```python
from build123d import *

# Parameters (mm, degrees)
BOX031_W     = 72
BOX031_H     = 58
BOX031_DEPTH = 4
FILLET025_R  = 10


with BuildPart() as fillet025:
    # Box031 → Box031 (new body)
    with BuildSketch(Plane(origin=(-15, -29, -2), x_dir=(1, 0, 0), z_dir=(0, 0, 1))):
        with Locations((36, 29)):
            Rectangle(BOX031_W, BOX031_H)
    extrude(amount=BOX031_DEPTH)

    # Fillet025
    fillet025_edges = [fillet025.edges().sort_by_distance(p)[0] for p in [
        (-15, -29, 0),
        (-15, 29, 0),
        (57, -29, 0),
        (57, 29, 0),
    ]]
    fillet(fillet025_edges, radius=FILLET025_R)


with BuildPart() as part_mirroring010:
    # Part__Mirroring010: instance of Fillet025
    add(fillet025.part.mirror(Plane(origin=(0, 0, 0), x_dir=(1, 0, 0), z_dir=(0, 1, 0))))


with BuildPart() as part_mirroring010_1:
    # Part__Mirroring010 placement: moved
    add(part_mirroring010.part.moved(Location((0, 72, 0))))


solid = part_mirroring010_1.part
```
Could you check a few things on this model? Use its own coordinates, in mm. Give positions to 0.01 mm unless a question says otherwise; leave off trailing zeros. Loops run counter-clockwise (first coordinate to the right, second up) from the corner with the lowest first, then second, coordinate; pieces in that order, holes last. Notation, with made-up numbers: (76, -15.5) - (110, -15.5) arc R22 ccw to (110, 23.5) - close; hole circle Ø7 at (-24, 87). An arc over 180 degrees is marked (long way). Answer in a Markdown table with one row per item. Add a question column.
Q1. If we section it at B-B (y = 47): List the corners of the cut face in (x, z) for me.
Q2. If we section it at A-A (z = -1.3): List the corners of the cut face in (x, y) for me.
Q3. We'd pull the mould along Y, two halves only. Please class faces 1 (the face through (-12.15, 97.99, 0.03)), 2 (the face through (-12.15, 46.01, 0.03)), 3 (the face through (20, 72, -2)): +Y half, -Y half, draft (parallel to the pull), parting line (faces both ways), or undercut.
Q4. If we section it at C-C (y = 94.5): List the corners of the cut face in (x, z) for me, plus the area to 3 significant figures.
Q5. Please list where these lines run through material, in increasing order: L1, parallel to X at y = 92.5, z = -0.85; L2, parallel to X at y = 50, z = 0.1. Write a range as from..to.
The answers:
| question | item | result |
|---|---|---|
| 1 | outline | (-13, -2) - (55, -2) - (55, 2) - (-13, 2) - close |
| 2 | outline | (-15, 53) arc R10 ccw to (-5, 43) - (47, 43) arc R10 ccw to (57, 53) - (57, 91) arc R10 ccw to (47, 101) - (-5, 101) arc R10 ccw to (-15, 91) - close |
| 3 | face 1 | +Y half |
| 3 | face 2 | -Y half |
| 3 | face 3 | draft |
| 4 | outline | (-14.37, -2) - (56.37, -2) - (56.37, 2) - (-14.37, 2) - close |
| 4 | area | 283 mm^2 |
| 5 | L1 | x = -14.89..56.89 |
| 5 | L2 | x = -14.54..56.54 |
